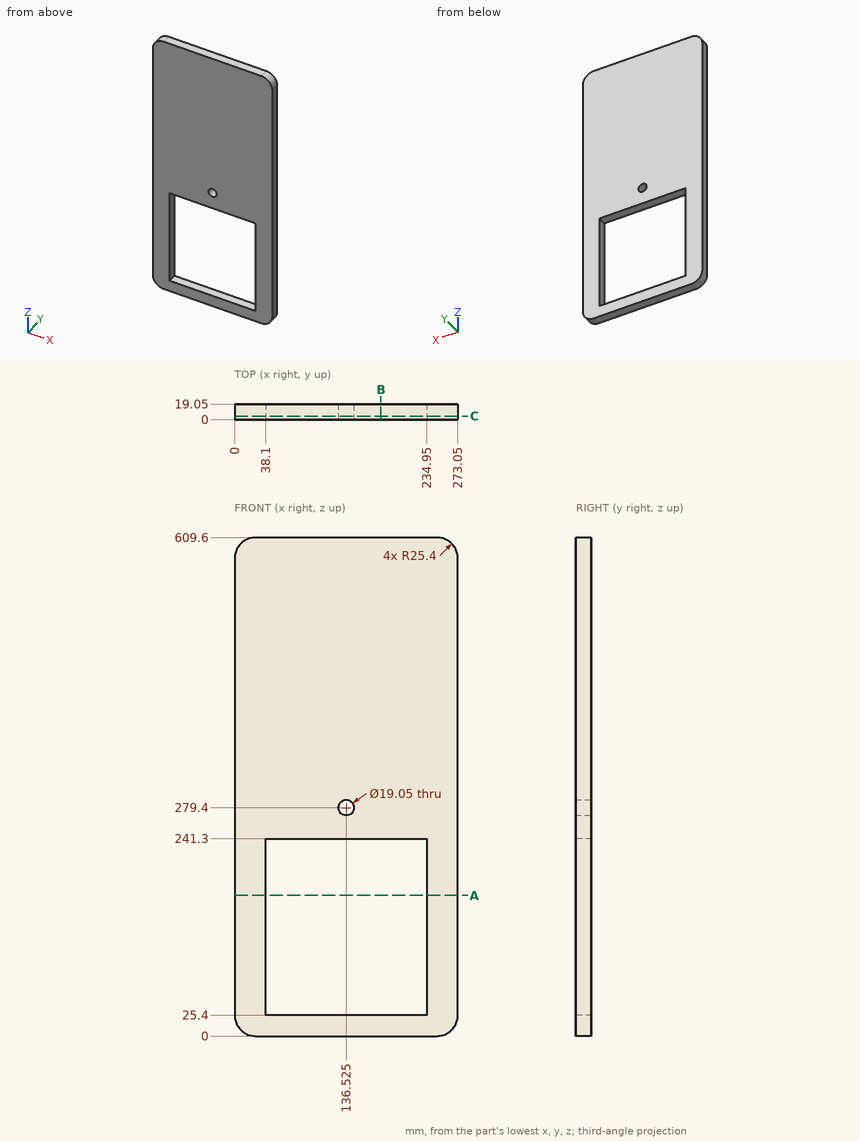
Geometry: see drawing. Coordinates: mm, zero at the bounding-box minimum. Give positions to 0.01 mm unless a question says otherwise; leave off trailing zeros. Write each loop counter-clockwise with the first axis right and the second up, starting at its lowest first coordinate (ties: lowest second). Pieces come first, ordered by that corner, then holes. Notation, with made-up numbers: (45.25, 55) -> (74.25, 55) arc R7 cw to (74.25, 68) -> close; hole circle Ø8 at (18, 58.25). An arc over 180 degrees is marked (long way). Use one line per item in the form item = value. Start each with the question number.
1) Ray query, probe 1 along Z at (x, y) = (82.5, 9.25); probe 2 along X at (y, z) = (15, 237.5); probe 3 along Z at (x, y) = (128, 18). Return the intervals inside material, ascending. Write a range as from..to.
2) Section query B-B on x = 179. Return the cut outline in (y, z).
3) Section query A-A on z = 172. Return the cut outline in (x, y).
4) Section query C-C on y = 4.25. Return the cut outline in (x, z) (3 decimals), then the cut area to 3 significant figures.
Outcome:
q1.probe_1 = 0..25.4, 241.3..609.6
q1.probe_2 = 0..38.1, 234.95..273.05
q1.probe_3 = 0..25.4, 241.3..275.15, 283.65..609.6
q2.outline = (0, 0) -> (19.05, 0) -> (19.05, 25.4) -> (0, 25.4) -> close; (0, 241.3) -> (19.05, 241.3) -> (19.05, 609.6) -> (0, 609.6) -> close
q3.outline = (0, 0) -> (38.1, 0) -> (38.1, 19.05) -> (0, 19.05) -> close; (234.95, 0) -> (273.05, 0) -> (273.05, 19.05) -> (234.95, 19.05) -> close
q4.outline = (0, 25.4) arc R25.4 ccw to (25.4, 0) -> (247.65, 0) arc R25.4 ccw to (273.05, 25.4) -> (273.05, 584.2) arc R25.4 ccw to (247.65, 609.6) -> (25.4, 609.6) arc R25.4 ccw to (0, 584.2) -> close; hole (38.1, 25.4) -> (234.95, 25.4) -> (234.95, 241.3) -> (38.1, 241.3) -> close; hole circle Ø19.05 at (136.525, 279.4)
q4.area = 123,000 mm^2
